Here's how the part is built. I have some questions about the finished solid (model axes, mm). Face numbers are marked on the shaded views. Round coordinates to 2 decimals unless told otherwise and drop trailing zeros. Write each loop counter-clockwise with the first axis right and the second up, starting at its lowest first coordinate (ties: lowest second). Pieces come first, ordered by that corner, then holes. Notation, with made-up numbers: (33.25, -5.75) - (72.25, -5.75) arc R13 ccw to (72.25, 19.25) - close; hole circle Ø11 at (69.5, -37.75). An arc over 180 degrees is marked (long way). Return JSON: item names as keys, results as strings. Group by question number.
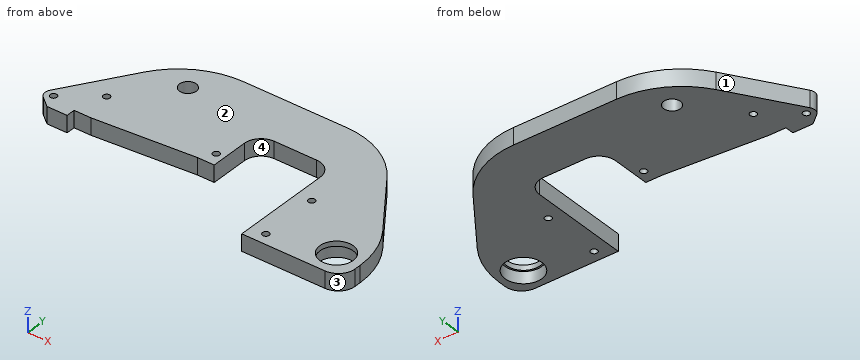
```python
from build123d import *

# Parameters (mm, degrees)
SKETCH1_R               = 11
SKETCH1_R_2             = 2
SKETCH1_W               = 10
SKETCH1_H               = 16
BOSS_EXTRUDE1_DEPTH     = 10
FILLET1_R               = 10
FILLET2_R               = 50
FILLET3_R               = 5
BOSS_EXTRUDE2_START     = -3
SKETCH2_R               = 11
SKETCH2_R_2             = 10
BOSS_EXTRUDE2_DEPTH     = 3
CUT_EXTRUDE1_DEPTH      = 124.835576471
CUT_EXTRUDE1_DEPTH_BACK = 124.835576471
SKETCH3_R               = 5


with BuildPart() as part:
    # Sketch1 → Boss-Extrude1 (new body)
    # profile 1 of 2: a face of its own
    with BuildSketch(Plane.XY):
        Polygon((-75, -13), (-65, -13), (-5, -8), (-5, 8), (5, 8), (5, 25), (50.5, 25), (50.5, -45), (76.132488073, -45), (110.5, -45), (110.5, -15), (60.5, 55), (-53.909617462, 55), (-96.658561066, -10.557288279), (-87.02, -18.32), (-75, -18.32), align=None)
        with Locations((95.5, -30)):
            Circle(SKETCH1_R, mode=Mode.SUBTRACT)
        with Locations((59.5, -38)):
            Circle(SKETCH1_R_2, mode=Mode.SUBTRACT)
        with Locations((59.5, -3)):
            Circle(SKETCH1_R_2, mode=Mode.SUBTRACT)
        with Locations((-70, 5.5)):
            Circle(SKETCH1_R_2, mode=Mode.SUBTRACT)
        with Locations((-90, -9.5)):
            Circle(SKETCH1_R_2, mode=Mode.SUBTRACT)
    # profile 2 of 2: a face of its own
    with BuildSketch(Plane.XY):
        Rectangle(SKETCH1_W, SKETCH1_H)
        Circle(SKETCH1_R_2, mode=Mode.SUBTRACT)
    extrude(amount=BOSS_EXTRUDE1_DEPTH)

    # Fillet1
    fillet1_edges = [part.edges().sort_by_distance(p)[0] for p in [
        (110.5, -45, 5),
        (50.5, 25, 5),
        (5, 25, 5),
    ]]
    fillet(fillet1_edges, radius=FILLET1_R)

    # Fillet2
    fillet2_edges = [part.edges().sort_by_distance(p)[0] for p in [
        (-53.909617462, 55, 5),
        (60.5, 55, 5),
        (110.5, -15, 5),
    ]]
    fillet(fillet2_edges, radius=FILLET2_R)

    # Fillet3
    fillet3_edges = [part.edges().sort_by_distance(p)[0] for p in [
        (-96.658561066, -10.557288279, 5),
    ]]
    fillet(fillet3_edges, radius=FILLET3_R)

    # Sketch2 → Boss-Extrude2 (add)
    with BuildSketch(Plane.XY.offset(10).offset(BOSS_EXTRUDE2_START)):
        with Locations((95.5, -30)):
            Circle(SKETCH2_R)
        with Locations((95.5, -30)):
            Circle(SKETCH2_R_2, mode=Mode.SUBTRACT)
    extrude(amount=BOSS_EXTRUDE2_DEPTH)

    # Sketch3 → Cut-Extrude1 (cut, two sides: drawn at the far end of the back side and taken through both)
    with BuildSketch(Plane.XY.offset(10).offset(-CUT_EXTRUDE1_DEPTH_BACK)):
        with Locations((-44.5, 35)):
            Circle(SKETCH3_R)
    extrude(amount=CUT_EXTRUDE1_DEPTH + CUT_EXTRUDE1_DEPTH_BACK, mode=Mode.SUBTRACT)


solid = part.part
```
1) Will these pins go through, and if not, where does the flat tip stop? pin 1 Ø2 at (x, z) = (-69, 2) entering from +Y; pin 2 Ø1.5 at (y, z) = (44.5, 8.5) entering from -X; pin 3 Ø1.5 at (y, z) = (-21, 5) entering from -X.
2) If we mould it in two halves opening along X, with no side actions, what happens to the marked faces 1, 2, 3 and 4? For each: released by +X, released by -X, zero draft, split by the parting line, or undercut.
3) Imagine slicing it at D-D (x = 59.5). Please give me the cut outline in (y, z).
4) Imagine slicing it at A-A (x = 0). Please give me the cut outline in (y, z), plus the area to 3 significant figures.
5) Imagine slicing it at C-C (y = 5.5). Please give me the cut outline in (x, z).
6) Imagine slicing it at B-B (z = 4.25). Please give me the cut outline in (x, y).
7) I need wall thicknesses on line 1 along Y through (x, z) = (59.5, 4.5); line 2 along X through (y, z) = (1, 9); line 3 along X through (y, z) = (13, 2.25). Which ranges of each line are inside material? Lowest first, please.
Results found:
{
 "1": {"pin 1": "stops at y = 33.36", "pin 2": "stops at x = -58.42", "pin 3": "stops at x = 50.5"},
 "2": {"face 1": "released by -X", "face 2": "zero draft", "face 3": "released by +X", "face 4": "undercut"},
 "3": {"outline": "(-45, 0) - (-40, 0) - (-40, 10) - (-45, 10) - close; (-36, 0) - (-5, 0) - (-5, 10) - (-36, 10) - close; (-1, 0) - (48.46, 0) - (48.46, 10) - (-1, 10) - close"},
 "4": {"outline": "(-8, 0) - (-2, 0) - (-2, 10) - (-8, 10) - close; (2, 0) - (55, 0) - (55, 10) - (2, 10) - close", "area": "590 mm²"},
 "5": {"outline": "(-86.19, 0) - (-72, 0) - (-72, 10) - (-86.19, 10) - close; (-68, 0) - (5, 0) - (5, 10) - (-68, 10) - close; (50.5, 0) - (95.86, 0) - (95.86, 10) - (50.5, 10) - close"},
 "6": {"outline": "(-94.19, -6.77) arc R5 ccw to (-93.14, -13.39) - (-87.02, -18.32) - (-75, -18.32) - (-75, -13) - (-65, -13) - (-5, -8) - (5, -8) - (5, 15) arc R10 cw to (15, 25) - (40.5, 25) arc R10 cw to (50.5, 15) - (50.5, -45) - (100.5, -45) arc R10 ccw to (110.5, -35) - (110.5, -31.02) arc R50 ccw to (101.19, -1.96) - (75.46, 34.06) arc R50 ccw to (34.77, 55) - (-26.82, 55) arc R50 ccw to (-68.7, 32.31) - close; hole circle Ø4 at (-90, -9.5); hole circle Ø4 at (-70, 5.5); hole circle Ø10 at (-44.5, 35); hole circle Ø4 at (0, 0); hole circle Ø4 at (59.5, -38); hole circle Ø4 at (59.5, -3); hole circle Ø22 at (95.5, -30)"},
 "7": {"line 1": "y = -45 to -40, -36 to -5, -1 to 48.46", "line 2": "x = -89.12 to -1.73, 1.73 to 5, 50.5 to 99.07", "line 3": "x = -81.3 to 5, 50.5 to 90.5"}
}
